Design review of the part shown in the three views and the two pictorial views. Dimensions are in mm from the part's minimum x, y and z. Round coordinates to 2 decimals unless told otherwise and drop trailing zeros. Loops run counter-clockwise (first coordinate to the right, second up) from the corner with the lowest first, then second, coordinate; pieces in that order, holes last. Notation, with made-up numbers: (-24, 84) - (15, 84) arc R16 ccw to (15, 96) - close; hole circle Ø10 at (11, 53.25). An arc over 180 degrees is marked (long way). Return JSON: item names as keys, results as strings. Group by question number.
(1) Wall thickness on L1, parallel to X at y = 8.5, z = 1.4 (1 decimal); L2, parallel to Y at x = 46, z = 2.5 (1 decimal); L3, parallel to X at y = 20, z = 1.15: over which ranges is each line inside the solid? List them lowest first. Write a range as [from, to].
(2) We need section B-B, the plane y = 6. Write out the cut boundary in (x, z), and give its area (3 significant figures).
(3) We need section D-D, the plane y = 31. Write out the cut boundary in (x, z).
(4) We need section A-A, the plane x = 44. Write out the cut boundary in (y, z).
(5) Clearance check with flat-ended pins moving along their axes: pin 1 (8 mm diameter, centred on x = 44, y = 6, fed in from +Z); pin 2 (1.5 mm diameter, centred on x = 16.5, z = 2, fed in from +Y). State where each tip first meets the part, or that it passes through.
(6) We need section C-C, the plane z = 1.25. Write out the cut boundary in (x, y).
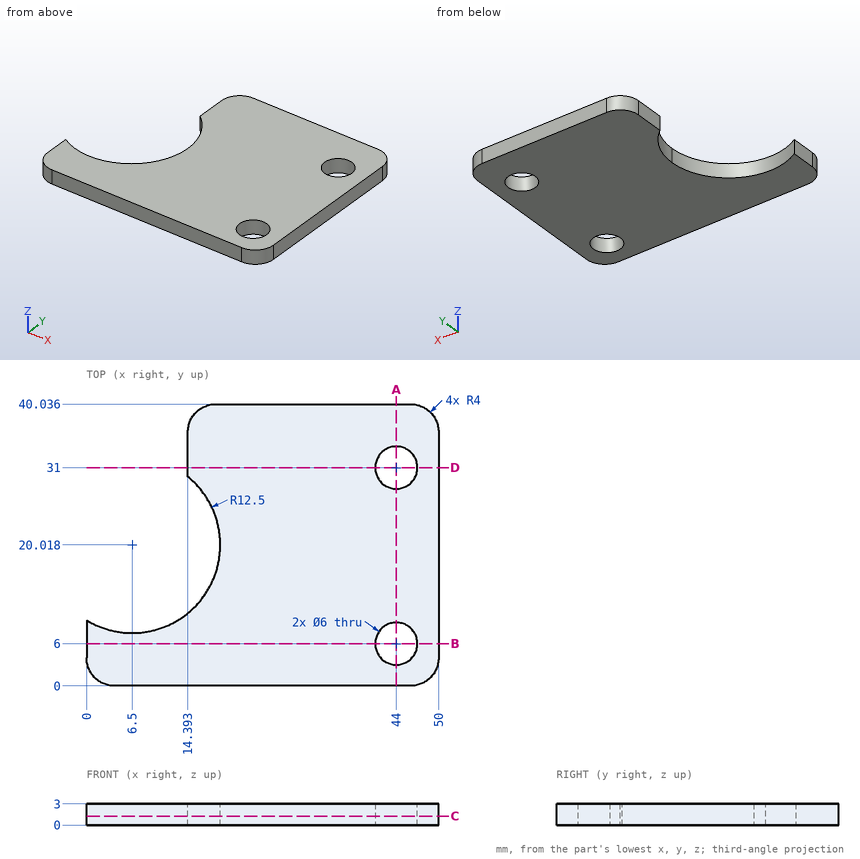
Solutions:
{
 "1": {"L1": "[0, 1.6], [11.4, 42.3], [45.7, 50]", "L2": "[0, 3.8], [8.2, 28.8], [33.2, 40]", "L3": "[19, 50]"},
 "2": {"outline": "(0, 0) - (41, 0) - (41, 3) - (0, 3) - close; (47, 0) - (50, 0) - (50, 3) - (47, 3) - close", "area": "132 mm^2"},
 "3": {"outline": "(14.39, 0) - (41, 0) - (41, 3) - (14.39, 3) - close; (47, 0) - (50, 0) - (50, 3) - (47, 3) - close"},
 "4": {"outline": "(0, 0) - (3, 0) - (3, 3) - (0, 3) - close; (9, 0) - (28, 0) - (28, 3) - (9, 3) - close; (34, 0) - (40.04, 0) - (40.04, 3) - (34, 3) - close"},
 "5": {"pin 1": "z = 3", "pin 2": "y = 39.87"},
 "6": {"outline": "(0, 4) arc R4 ccw to (4, 0) - (46, 0) arc R4 ccw to (50, 4) - (50, 36.04) arc R4 ccw to (46, 40.04) - (18.39, 40.04) arc R4 ccw to (14.39, 36.04) - (14.39, 29.71) arc R12.5 cw to (0, 9.34) - close; hole circle Ø6 at (44, 6); hole circle Ø6 at (44, 31)"}
}
